from build123d import *

# Parameters (mm, degrees)
BOSS_EXTRU_1_DEPTH      = 3
CONG_1_R                = 5
ESQUISSE2_R             = 1
ESQUISSE2_R_2           = 1.5
ENL_V_MAT_EXTRU_2_DEPTH = 3
D_GAGEMENT_M31_D        = 3.4
D_GAGEMENT_M31_DEPTH    = 10
D_GAGEMENT_M31_TIP      = 1.021463052


with BuildPart() as part:
    # Esquisse1 → Boss.-Extru.1 (new body)
    with BuildSketch(Plane(origin=(0, 0, 0), x_dir=(1, 0, 0), z_dir=(0, 1, 0))):
        Polygon((-67.5, 0), (67.5, 0), (67.5, 30), (15, 75), (-15, 75), (-67.5, 75), (-67.5, 30), align=None)
    extrude(amount=BOSS_EXTRU_1_DEPTH)

    # Congé1
    cong_1_edges = [part.edges().sort_by_distance(p)[0] for p in [
        (67.5, 1.5, 0),
        (-67.5, 1.5, 0),
        (-67.5, 1.5, -75),
        (15, 1.5, -75),
        (67.5, 1.5, -30),
    ]]
    fillet(cong_1_edges, radius=CONG_1_R)

    # Esquisse2 → Enlèv. mat.-Extru.2 (cut)
    with BuildSketch(Plane(origin=(0, 3, 0), x_dir=(1, 0, 0), z_dir=(0, 1, 0))):
        with Locations(Location((-62.5, 5, 0), (0, 0, 270))):
            Circle(ESQUISSE2_R)
        with Locations(Location((62.5, 5, 0), (0, 0, 270))):
            Circle(ESQUISSE2_R)
        with Locations(Location((0, 70, 0), (0, 0, 270))):
            Circle(ESQUISSE2_R)
        with Locations(Location((-58.5, 15.99, 0), (0, 0, 270))):
            Circle(ESQUISSE2_R_2)
        with Locations(Location((-58.5, 50, 0), (0, 0, 270))):
            Circle(ESQUISSE2_R_2)
        with Locations(Location((-38.5, 70, 0), (0, 0, 270))):
            Circle(ESQUISSE2_R_2)
        with Locations(Location((48.5, 39.85, 0), (0, 0, 270))):
            Circle(ESQUISSE2_R_2)
    extrude(amount=-ENL_V_MAT_EXTRU_2_DEPTH, mode=Mode.SUBTRACT)

    # Dégagement M31
    with Locations(Plane(origin=(0, 3, 0), x_dir=(1, 0, 0), z_dir=(0, 1, 0))):
        with Locations((-62.5, 5), (62.5, 5), (0, 70), (-58.5, 15.99), (-58.5, 50), (-38.5, 70), (48.5, 39.85)):
            Hole(D_GAGEMENT_M31_D / 2, depth=D_GAGEMENT_M31_DEPTH)
            with Locations((0, 0, -(D_GAGEMENT_M31_DEPTH + D_GAGEMENT_M31_TIP / 2))):  # 118° drill point
                Cone(0, D_GAGEMENT_M31_D / 2, D_GAGEMENT_M31_TIP, mode=Mode.SUBTRACT)


solid = part.part
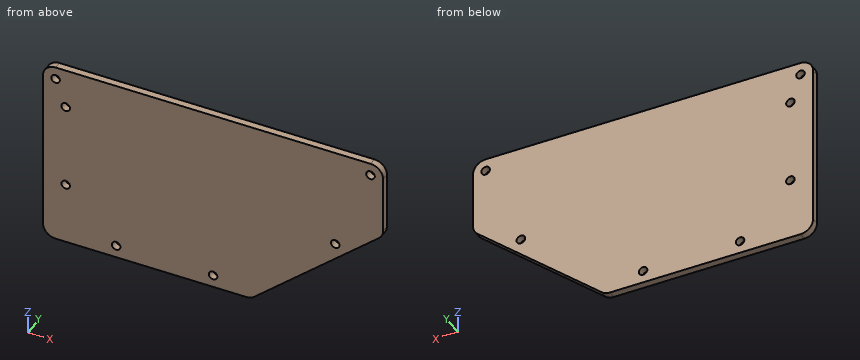
Source: CAD feature listing. Evaluate the final solid. Frame: model axes, mm. Round coordinates to 2 decimals unless told otherwise and drop trailing zeros. Order: outer loops, then holes, each group sorted by start corner. A loop starts at its lowest first (then second) coordinate and runs counter-clockwise, first axis right, second up. Notation, with made-up numbers: (59, 72.25) -> (90, 72.25) arc R23 ccw to (90, 111.25) -> close; hole circle Ø8 at (8, 62.5). An arc over 180 degrees is marked (long way). Answer as CSV lines item,"result".
Item 1: Section C-C, the plane y = 1.45. Return loops of the section in (x, z).
A:
outline,"(-67.5, -70) arc R5 ccw to (-62.5, -75) -> (13.15, -75) arc R5 ccw to (16.4, -73.8) -> (65.75, -31.5) arc R5 ccw to (67.5, -27.7) -> (67.5, -5) arc R5 ccw to (62.5, 0) -> (-62.5, 0) arc R5 ccw to (-67.5, -5) -> close; hole circle Ø3.4 at (-62.5, -5); hole circle Ø3.4 at (-58.5, -50); hole circle Ø3.4 at (-58.5, -15.99); hole circle Ø3.4 at (-38.5, -70); hole circle Ø3.4 at (0, -70); hole circle Ø3.4 at (48.5, -39.85); hole circle Ø3.4 at (62.5, -5)"
Item 2: Line query: L1, parallel to Z at x = -62.5, y = 1.1; L2, parallel to Z at x = -38.5, y = 1.85; L3, parallel to X at y = 0.7, z = -68.5. Output: solid intervals per line, ascending.
A:
L1,"-75 to -6.7, -3.3 to 0"
L2,"-75 to -71.7, -68.3 to 0"
L3,"-67.5 to -39.3, -37.7 to -0.8, 0.8 to 22.58"
Item 3: Pin query (flat end, axial travel): pin 1 Ø1.5 at (y, z) = (1, -50.5) entering from +X; pin 2 Ø3 at (x, z) = (-62.5, -5) entering from +Y. Return the tip coordinate at first contact, or that it passes through.
A:
pin 1,"x = 44.46"
pin 2,"through"
Item 4: Section B-B, the plane z = -39.85. Return loops of the section in (x, y).
A:
outline,"(-67.5, 0) -> (46.8, 0) -> (46.8, 3) -> (-67.5, 3) -> close; (50.2, 0) -> (56.01, 0) -> (56.01, 3) -> (50.2, 3) -> close"
Item 5: Section D-D, the plane x = 40. Return loops of the section in (y, z).
A:
outline,"(0, -53.57) -> (3, -53.57) -> (3, 0) -> (0, 0) -> close"
Item 6: Section A-A, the plane x = 0. Return loops of the section in (y, z), plus the area to 3 significant figures.
A:
outline,"(0, -75) -> (3, -75) -> (3, -71.7) -> (0, -71.7) -> close; (0, -68.3) -> (3, -68.3) -> (3, 0) -> (0, 0) -> close"
area,"215 mm²"
